```python
from build123d import *

# Parameters (mm, degrees)
BOSS_EXTRU_1_DEPTH = 13.4
ESQUISSE2_R        = 5.805
BOSS_EXTRU_2_DEPTH = 10
ESQUISSE3_R        = 3.5
BOSS_EXTRU_3_DEPTH = 4
ESQUISSE4_R        = 4.25
BOSS_EXTRU_4_DEPTH = 6.45


with BuildPart() as part:
    # Esquisse1 → Boss.-Extru.1 (new body)
    with BuildSketch(Plane.XY):
        with BuildLine():
            Line((-6.65, 0), (-6.65, -23.65))
            Line((-6.65, -23.65), (6.65, -23.65))
            Line((6.65, -23.65), (6.65, 0))
            ThreePointArc((6.65, 0), (0, 6.65), (-6.65, 0))
        make_face()
    extrude(amount=BOSS_EXTRU_1_DEPTH)

    # Esquisse2 → Boss.-Extru.2 (add)
    with BuildSketch(Plane(origin=(0, 0, 0), x_dir=(-1, 0, 0), z_dir=(0, 0, -1))):
        with Locations((0, -3.665)):
            Circle(ESQUISSE2_R)
    extrude(amount=BOSS_EXTRU_2_DEPTH)

    # Esquisse3 → Boss.-Extru.3 (add)
    with BuildSketch(Plane(origin=(0, 0, -10), x_dir=(-1, 0, 0), z_dir=(0, 0, -1))):
        with Locations((0, -3.665)):
            Circle(ESQUISSE3_R)
    extrude(amount=BOSS_EXTRU_3_DEPTH)

    # Esquisse4 → Boss.-Extru.4 (add)
    with BuildSketch(Plane(origin=(0, 0, -14), x_dir=(-1, 0, 0), z_dir=(0, 0, -1))):
        with Locations((0, -3.665)):
            Circle(ESQUISSE4_R)
    extrude(amount=BOSS_EXTRU_4_DEPTH)


solid = part.part
```
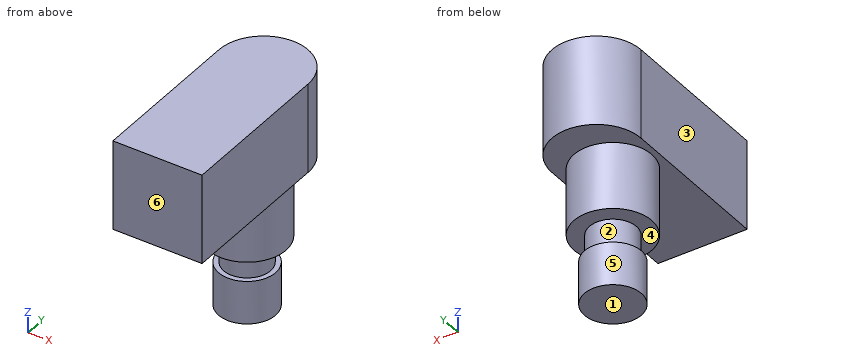
Verification items for the finished model (mm, model axes). Face numbers are marked on the shaded views. A direction names the side the tool comes from. Coordinates: 2 decimals unless noted, no trailing zeros. Loops run counter-clockwise (first coordinate to the right, second up) from the corner with the lowest first, then second, coordinate; pieces in that order, holes last. Notation, with made-up numbers: (-4, -17.75) -> (33, -17.75) arc R30 ccw to (33, 8.25) -> close; hole circle Ø3 at (60.5, -26.5). An arc over 180 degrees is marked (long way). Answer in a Markdown table with one row per item. Add a question column.
1. Access from +Z, -Z, +X, -X, +Y, -Y to the whole of each face (thin tool, end or side, straight path). Record for the marked faces 4, 5 and 6.
2. Material ranges on probe 1 along Z at (x, y) = (-4, -2.5); probe 2 along X at (y, z) = (-3.5, -8); probe 3 along Z at (x, y) = (3.25, -15), recorded low to high. Write a range as [from, to].
3. Section check A-A, the plane x = 0. Enter the section's corners in (y, z) (3 decimals).
4. Depth check by flat-ended pin: P1, Ø1, axis at x = 4, z = -16.5, coming from the +Y side; P2, Ø6, axis at x = -2, y = -14, coming from the -Z side. Enter the tip coordinate at first touch or a pass-through.
5. Draft check along Z on the marked faces 1, 2 and 3. Enter one of: +Z half, -Z half, draft (parallel to the pull), parting line (faces both ways), or undercut.
6. Section check C-C, the plane z = 5. Enter the section's corners in (x, y).
7. Section check D-D, the plane y = -19. Enter the section's corners in (x, z).
8. Section check B-B, the plane y = -6. Enter the section's corners in (x, z), then the cut area to 3 significant figures.
Derived:
| question | item | result |
|---|---|---|
| 1 | face 4 | none |
| 1 | face 5 | -Z |
| 1 | face 6 | +Z, -Z, +X, -X, -Y |
| 2 | probe 1 | z = [-20.45, -14], [-10, 13.4] |
| 2 | probe 2 | x = [-5.8, 5.8] |
| 2 | probe 3 | z = [0, 13.4] |
| 3 | outline | (-23.65, 0) -> (-9.47, 0) -> (-9.47, -10) -> (-7.165, -10) -> (-7.165, -14) -> (-7.915, -14) -> (-7.915, -20.45) -> (0.585, -20.45) -> (0.585, -14) -> (-0.165, -14) -> (-0.165, -10) -> (2.14, -10) -> (2.14, 0) -> (6.65, 0) -> (6.65, 13.4) -> (-23.65, 13.4) -> close |
| 4 | P1 | stops at y = -1.25 |
| 4 | P2 | stops at z = 0 |
| 5 | face 1 | -Z half |
| 5 | face 2 | undercut |
| 5 | face 3 | draft |
| 6 | outline | (-6.65, -23.65) -> (6.65, -23.65) -> (6.65, 0) arc R6.65 ccw to (-6.65, 0) -> close |
| 7 | outline | (-6.65, 0) -> (6.65, 0) -> (6.65, 13.4) -> (-6.65, 13.4) -> close |
| 8 | outline | (-6.65, 0) -> (-5.31, 0) -> (-5.31, -10) -> (-2.61, -10) -> (-2.61, -14) -> (-3.55, -14) -> (-3.55, -20.45) -> (3.55, -20.45) -> (3.55, -14) -> (2.61, -14) -> (2.61, -10) -> (5.31, -10) -> (5.31, 0) -> (6.65, 0) -> (6.65, 13.4) -> (-6.65, 13.4) -> close |
| 8 | area | 351 mm² |
